from build123d import *

# Parameters (mm, degrees)
F2_W     = 13.8
F2_H     = 6
F6_W     = 12.6
F6_H     = 4.4
F8_W     = 15.8
F8_H     = 8
F9_DEPTH = 4
F10_SIZE = 0.99999


# Not quite as in the source:
# - a fillet or chamfer is up to 0.001 mm smaller than in the source, because OpenCascade refuses the exact size
# - the arcs of a loft's sections are written as splines that run evenly, so that the points pair up as in the source's solid


with BuildPart() as f3:
    # F0 (on Top) → F3 section 0
    with BuildSketch(Plane.XY):
        with BuildLine():
            add(Edge.make_bspline(
                [(-6.3277833881, 2.7512101688), (-6.6879159571, 1.9229052602), (-6.883211565, 1.0233196176), (-6.914692653, -0.782821821), (-6.7508657466, -1.6886669775), (-6.0887700743, -3.3693713762), (-5.5907618149, -4.143569333), (-4.3358874467, -5.4429646828), (-3.5795150773, -5.9676508192), (-2.7512101688, -6.3277833881)],
                knots=[0, 0, 0, 0, 0.25, 0.25, 0.5, 0.5, 0.75, 0.75, 1, 1, 1, 1], degree=3))
            add(Edge.make_bspline(
                [(-2.7512101688, -6.3277833881), (-1.9229052602, -6.6879159571), (-1.0233196176, -6.883211565), (0.782821821, -6.914692653), (1.6886669775, -6.7508657466), (3.3693713762, -6.0887700743), (4.143569333, -5.5907618149), (5.4429646828, -4.3358874467), (5.9676508192, -3.5795150773), (6.3277833881, -2.7512101688)],
                knots=[0, 0, 0, 0, 0.25, 0.25, 0.5, 0.5, 0.75, 0.75, 1, 1, 1, 1], degree=3))
            add(Edge.make_bspline(
                [(6.3277833881, -2.7512101688), (6.6879159571, -1.9229052602), (6.883211565, -1.0233196176), (6.914692653, 0.782821821), (6.7508657466, 1.6886669775), (6.0887700743, 3.3693713762), (5.5907618149, 4.143569333), (4.3358874467, 5.4429646828), (3.5795150773, 5.9676508192), (2.7512101688, 6.3277833881)],
                knots=[0, 0, 0, 0, 0.25, 0.25, 0.5, 0.5, 0.75, 0.75, 1, 1, 1, 1], degree=3))
            add(Edge.make_bspline(
                [(2.7512101688, 6.3277833881), (1.9229052602, 6.6879159571), (1.0233196176, 6.883211565), (-0.782821821, 6.914692653), (-1.6886669775, 6.7508657466), (-3.3693713762, 6.0887700743), (-4.143569333, 5.5907618149), (-5.4429646828, 4.3358874467), (-5.9676508192, 3.5795150773), (-6.3277833881, 2.7512101688)],
                knots=[0, 0, 0, 0, 0.25, 0.25, 0.5, 0.5, 0.75, 0.75, 1, 1, 1, 1], degree=3))
        make_face()
    # F2 (on offset) → F3 section 1
    with BuildSketch(Plane.XY.offset(40)):
        Rectangle(F2_W, F2_H)
    loft(ruled=True)

    # F5 (on Top) → F7 section 0
    with BuildSketch(Plane.XY):
        with BuildLine():
            add(Edge.make_bspline(
                [(-5.947778016, 2.0770018469), (-6.219656922, 1.2984395252), (-6.3366241137, 0.4661247359), (-6.2431050237, -1.1805579575), (-6.0326555377, -1.9942779624), (-5.3160969794, -3.479826193), (-4.8102698423, -4.151069919), (-3.5797613606, -5.2493224353), (-2.8555641686, -5.6758991101), (-2.0770018469, -5.947778016)],
                knots=[0, 0, 0, 0, 0.25, 0.25, 0.5, 0.5, 0.75, 0.75, 1, 1, 1, 1], degree=3))
            add(Edge.make_bspline(
                [(-2.0770018469, -5.947778016), (-1.2984395252, -6.219656922), (-0.4661247359, -6.3366241137), (1.1805579575, -6.2431050237), (1.9942779624, -6.0326555377), (3.479826193, -5.3160969794), (4.151069919, -4.8102698423), (5.2493224353, -3.5797613606), (5.6758991101, -2.8555641686), (5.947778016, -2.0770018469)],
                knots=[0, 0, 0, 0, 0.25, 0.25, 0.5, 0.5, 0.75, 0.75, 1, 1, 1, 1], degree=3))
            add(Edge.make_bspline(
                [(5.947778016, -2.0770018469), (6.219656922, -1.2984395252), (6.3366241137, -0.4661247359), (6.2431050237, 1.1805579575), (6.0326555377, 1.9942779624), (5.3160969794, 3.479826193), (4.8102698423, 4.151069919), (3.5797613606, 5.2493224353), (2.8555641686, 5.6758991101), (2.0770018469, 5.947778016)],
                knots=[0, 0, 0, 0, 0.25, 0.25, 0.5, 0.5, 0.75, 0.75, 1, 1, 1, 1], degree=3))
            add(Edge.make_bspline(
                [(2.0770018469, 5.947778016), (1.2984395252, 6.219656922), (0.4661247359, 6.3366241137), (-1.1805579575, 6.2431050237), (-1.9942779624, 6.0326555377), (-3.479826193, 5.3160969794), (-4.151069919, 4.8102698423), (-5.2493224353, 3.5797613606), (-5.6758991101, 2.8555641686), (-5.947778016, 2.0770018469)],
                knots=[0, 0, 0, 0, 0.25, 0.25, 0.5, 0.5, 0.75, 0.75, 1, 1, 1, 1], degree=3))
        make_face()
    # F6 (on offset) → F7 section 1
    with BuildSketch(Plane.XY.offset(38)):
        Rectangle(F6_W, F6_H)
    loft(ruled=True, mode=Mode.SUBTRACT)

    # F8 (on offset) → F9 (join)
    with BuildSketch(Plane.XY.offset(40)):
        Rectangle(F8_W, F8_H)
    extrude(amount=F9_DEPTH)

    # F10 (size 1 in the source; OpenCascade refuses exactly that, so slightly less here)
    f10_edges = [f3.edges().sort_by_distance(p)[0] for p in [
        (7.9, 0, 44),
        (0, -4, 44),
        (0, 4, 44),
        (-7.9, 0, 44),
        (0, -4, 40),
        (-7.9, 0, 40),
        (0, 4, 40),
        (7.9, 0, 40),
    ]]
    chamfer(f10_edges, length=F10_SIZE)


solid = f3.part
Can you work these out from the model? Positions are in its coordinate system, mm. A direction names the side the tool comes from. Coordinates: 2 decimals unless noted, no trailing zeros. Loops run counter-clockwise (first coordinate to the right, second up) from the corner with the lowest first, then second, coordinate; pieces in that order, holes last. Notation, with made-up numbers: (38, 51) - (52, 51) arc R14 cw to (52, 57) - close; hole circle Ø3 at (78, 2.25). An arc over 180 degrees is marked (long way). Answer as a JSON object with one key per item and string values. Group by question number.
Item 1: If we section it at A-A (z = 40.5): List the corners of the cut face in (x, y) for me, plus the area to 3 significant figures.
Item 2: If we mould it in two halves opening along Z, with no side actions, what happens to faces 4 (the face through (-0.1, 3.5, 40.5)), 5 (the face through (0, -4, 42)), 6 (the face through (-7.4, -0.1, 40.5)), 7 (the face through (-0.1, -3.5, 43.5))? For each: released by +Z, released by -Z, zero draft, split by the parting line, or undercut.
Item 3: For pin 1 (3 mm diameter, centred on x = -1.5, y = 0.5, fed in from -Z); pin 2 (6 mm diameter, centred on x = 2.5, y = -5, fed in from -Z); pin 3 (1.5 mm diameter, centred on x = 4, z = 10.5, fed in from -Y); pin 4 (1.6 mm diameter, centred on x = -2.5, z = 41.5, fed in from -Y), each with a flat end and sliding along its axis, tell me the tip position at first contact or that it passes through.
Item 4: If I drill on L1, parallel to Z at x = 2.75, y = -0.75; L2, parallel to Y at x = -2.5, z = 36; L3, parallel to Y at x = -1.5, z = 41.5, over which ranges is the centre line in solid material (lowest first)? Write a range as from..to.
Item 5: On a 3-axis mill with a long thin cutter (end or side, diameter ignored), from which of +Z, -Z, +X, -X, +Y, -Y can I reach the whole of each face in a straight line? I mean faces 1 (the face through (0, 4, 42)), 2 (the face through (7.4, -0.1, 43.5)), 3 (the face through (-0.1, -3.5, 40.5)). Say none if no direction works.
Returned:
{
 "1": {"outline": "(-7.4, -3.5) - (7.4, -3.5) - (7.4, 3.5) - (-7.4, 3.5) - close", "area": "104 mm²"},
 "2": {"face 4": "undercut", "face 5": "zero draft", "face 6": "released by -Z", "face 7": "released by +Z"},
 "3": {"pin 1": "stops at z = 38", "pin 2": "stops at z = 0", "pin 3": "stops at y = -5.06", "pin 4": "stops at y = -4"},
 "4": {"L1": "z = 38..44", "L2": "y = -3.39..-2.41, 2.33..3.25", "L3": "y = -4..4"},
 "5": {"face 1": "+Z, +X, -X, +Y", "face 2": "+Z, +X, +Y, -Y", "face 3": "+X, -X, -Y"}
}
